For this review, take the finished solid that the model builds, in its own axes (mm). Give positions to 0.01 mm unless a question says otherwise; leave off trailing zeros. Use CSV: the item, a comma, the result in double quotes. Start each with the question number.
1. Wall thickness on line 1 (Y direction, x = 12, z = 24.5): over which ranges is the line inside the solid? List them lowest first.
2. Mouldability with a two-part tool opening along X and no side actions: class faces 1 (the flat face through (25.456, 0.887, 15.21)), 2 (the flat face through (65.67, 0.89, 15.21)), 3 (the flat face through (45.562, 0.887, 15.21)) as pulls with the +X half, pulls with the -X half, needs draft (parallel to the pull), parting line crosses it, or undercut.
3. For pin 1 (1.5 mm diameter, centred on x = 54.5, z = 19.5, fed in from +Y); pin 2 (12 mm diameter, centred on x = 15, z = 24.5, fed in from +Y), all flat-tipped, find the tip position at first contact; note any pin that passes through.
```python
from build123d import *

# Parameters (mm, degrees)
SKETCH1_W           = 85.451320178
SKETCH1_H           = 8
EXTRUDE1_DEPTH      = 30
EXTRUDE2_DEPTH      = 30
LPATTERN1_COUNT     = 34
LPATTERN1_PITCH     = 2.513274123
SKETCH_1_W          = 24.951320178
SKETCH_1_H          = 8.70222752
CUT_EXTRUDE_1_DEPTH = 40


with BuildPart() as part:
    # Sketch1 → Extrude1 (new body)
    with BuildSketch(Plane.XY):
        with Locations((42.725660089, -4)):
            Rectangle(SKETCH1_W, SKETCH1_H)
    extrude(amount=EXTRUDE1_DEPTH)

    # Sketch2 → Extrude2 (add)
    with BuildSketch(Plane.XY.offset(30)):
        Polygon((0, 0), (0.655146422, 1.8), (1.329431108, 1.8), (1.98457753, 0), align=None)
    extrude2 = extrude(amount=-EXTRUDE2_DEPTH)

    # LPattern1: Extrude2 ×34
    with Locations(*[(i * LPATTERN1_PITCH, 0, 0) for i in range(1, LPATTERN1_COUNT)]):
        add(extrude2)

    # 草图1 → 切除-拉伸1 (cut)
    with BuildSketch(Plane.XY.offset(30)):
        with Locations((12.475660089, 4.35111376)):
            Rectangle(SKETCH_1_W, SKETCH_1_H)
    extrude(amount=-CUT_EXTRUDE_1_DEPTH, mode=Mode.SUBTRACT)


solid = part.part
```
Check result:
1,line 1,"y = -8 to 0"
2,face 1,"pulls with the -X half"
2,face 2,"undercut"
2,face 3,"undercut"
3,pin 1,"stops at y = 1.8"
3,pin 2,"stops at y = 0"
